Source: three-view drawing plus pictorial views. Frame: mm from the lowest corner of the part. A direction names the side the tool comes from. Coordinates: 2 decimals unless noted, no trailing zeros. Loops run counter-clockwise (first coordinate to the right, second up) from the corner with the lowest first, then second, coordinate; pieces in that order, holes last. Notation, with made-up numbers: (25, -4) -> (81, -4) arc R28 ccw to (81, 14) -> close; hole circle Ø11 at (2.25, 17). An arc over 180 degrees is marked (long way). Answer as a JSON object with one key per item and string values. Group by question number.
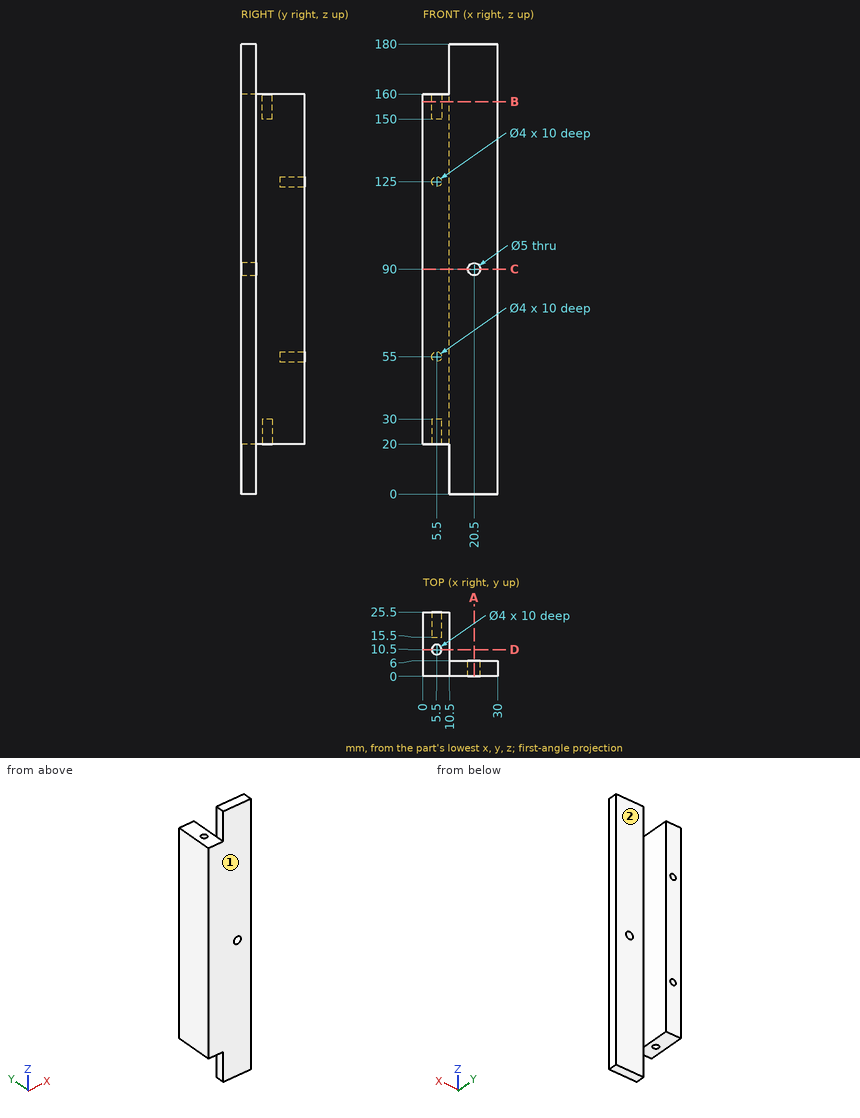
1. Section query D-D on y = 10.5. Return loops of the section in (x, z), then the cut area to 3 significant figures.
2. Section query C-C on z = 90. Return loops of the section in (x, y), then the cut area to 3 significant figures.
3. Section query A-A on x = 20.5. Return loops of the section in (y, z).
4. Pin query (flat end, axial travel): pin 1 Ø1.5 at (y, z) = (17, 123.5) entering from +X; pin 2 Ø12 at (x, y) = (24, 13.5) entering from +Z; pin 3 Ø4.5 at (x, y) = (5.5, 10.5) entering from +Z; pin 4 Ø2 at (x, z) = (21.5, 35.5) entering from +Y. Return the tip coordinate at first contact, or that it passes through.
5. Section query B-B on z = 157. Return loops of the section in (x, y), then the cut area to 3 significant figures.
6. Reachability of the marked faces 1 and 2 from +Z, -Z, +X, -X, +Y, -Y: full face, straight path, thin tool, end or side. Return the list, or none.
7. Ray query, L1, parallel to Z at x = 5.5, y = 22.75; L2, parallel to Y at x = 5.5, z = 153.25; L3, parallel to Z at x = 5, y = 24.75. Return the intervals inside material, ascending.
Solved:
{
 "1": {"outline": "(0, 20) -> (3.5, 20) -> (3.5, 30) -> (7.5, 30) -> (7.5, 20) -> (10.5, 20) -> (10.5, 160) -> (7.5, 160) -> (7.5, 150) -> (3.5, 150) -> (3.5, 160) -> (0, 160) -> close", "area": "1,390 mm^2"},
 "2": {"outline": "(0, 0) -> (18, 0) -> (18, 6) -> (10.5, 6) -> (10.5, 25.5) -> (0, 25.5) -> close; (23, 0) -> (30, 0) -> (30, 6) -> (23, 6) -> close", "area": "355 mm^2"},
 "3": {"outline": "(0, 0) -> (6, 0) -> (6, 87.5) -> (0, 87.5) -> close; (0, 92.5) -> (6, 92.5) -> (6, 180) -> (0, 180) -> close"},
 "4": {"pin 1": "x = 10.5", "pin 2": "through", "pin 3": "z = 160", "pin 4": "y = 6"},
 "5": {"outline": "(0, 0) -> (30, 0) -> (30, 6) -> (10.5, 6) -> (10.5, 25.5) -> (0, 25.5) -> close; hole circle Ø4 at (5.5, 10.5)", "area": "372 mm^2"},
 "6": {"face 1": "+Z, -Z, +X, -X, -Y", "face 2": "+Z, -Z, +X, +Y"},
 "7": {"L1": "20 to 53, 57 to 123, 127 to 160", "L2": "0 to 8.5, 12.5 to 25.5", "L3": "20 to 53.06, 56.94 to 123.06, 126.94 to 160"}
}
